For this review, take the finished solid that the model builds, in its own axes (mm). A direction names the side the tool comes from. Give positions to 0.01 mm unless a question says otherwise; leave off trailing zeros. Write each loop counter-clockwise with the first axis right and the second up, starting at its lowest first coordinate (ties: lowest second). Pieces come first, ordered by that corner, then holes. Notation, with made-up numbers: (7, 75.25) -> (27, 75.25) arc R13 cw to (27, 92.25) -> close; hole circle Ø7 at (60.25, 53). An arc over 180 degrees is marked (long way). Answer as CSV lines item,"result".
```python
from build123d import *

# Parameters (mm, degrees)
SKETCH2_R            = 215
SKETCH2_R_2          = 190
SKETCH2_R_3          = 155
BOSS_EXTRUDE1_DEPTH  = 390
SKETCH2_3_R          = 155
SKETCH2_3_R_2        = 125
BOSS_EXTRUDE2_DEPTH  = 315
SKETCH2_5_R          = 125
SKETCH2_5_R_2        = 105
SKETCH2_5_R_3        = 80
BOSS_EXTRUDE4_DEPTH  = 190
SKETCH2_6_R          = 125
SKETCH2_6_R_2        = 105
SKETCH2_6_R_3        = 80
CUT_EXTRUDE1_DEPTH   = 165
SKETCH2_7_R          = 125
SKETCH2_7_R_2        = 105
BOSS_EXTRUDE5_DEPTH  = 165
CUT_EXTRUDE2_START   = -165
SKETCH2_9_R          = 105
CUT_EXTRUDE2_DEPTH   = 165
CUT_EXTRUDE2_DRAFT   = -8.7461623
SKETCH2_10_R         = 155
SKETCH2_10_R_2       = 125
BOSS_EXTRUDE6_DEPTH  = 165
SKETCH2_12_R         = 215
SKETCH2_12_R_2       = 190
CUT_EXTRUDE3_DEPTH   = 60
SKETCH2_13_R         = 290
SKETCH2_13_R_2       = 190
SKETCH2_13_R_3       = 125
SKETCH2_13_R_4       = 80
BOSS_EXTRUDE7_DEPTH  = 35
BOSS_EXTRUDE8_START  = 100
SKETCH3_R            = 190
SKETCH3_R_2          = 175
SKETCH3_R_3          = 155
SKETCH3_R_4          = 125
BOSS_EXTRUDE8_DEPTH  = 100
BOSS_EXTRUDE10_START = 150
SKETCH3_5_R          = 175
SKETCH3_5_R_2        = 155
SKETCH3_5_R_3        = 125
BOSS_EXTRUDE10_DEPTH = 150
BOSS_EXTRUDE11_START = 250
SKETCH3_6_R          = 155
SKETCH3_6_R_2        = 125
BOSS_EXTRUDE11_DEPTH = 250
CUT_EXTRUDE5_REACH   = 567.951
SKETCH4_R            = 24
CIRPATTERN2_COUNT    = 8
SKETCH6_W            = 22
SKETCH6_H            = 75
BOSS_EXTRUDE12_DEPTH = 12.5
CIRPATTERN3_COUNT    = 8


with BuildPart() as part:
    # Sketch2 → Boss-Extrude1 (new body)
    # profile 1 of 2: a face of its own
    with BuildSketch(Plane(origin=(0, 0, 0), x_dir=(0, 1, 0), z_dir=(0, 0, 1))):
        with Locations(Location((0, 0, 0), (0, 0, 270))):
            Circle(SKETCH2_R)
        Circle(SKETCH2_R_2, mode=Mode.SUBTRACT)
    # profile 2 of 2: a face of its own
    with BuildSketch(Plane(origin=(0, 0, 0), x_dir=(0, 1, 0), z_dir=(0, 0, 1))):
        Circle(SKETCH2_R_2)
        with Locations(Location((0, 0, 0), (0, 0, 270))):
            Circle(SKETCH2_R_3, mode=Mode.SUBTRACT)
    extrude(amount=-BOSS_EXTRUDE1_DEPTH)

    # Sketch2_3 → Boss-Extrude2 (add)
    with BuildSketch(Plane(origin=(0, 0, 0), x_dir=(0, 1, 0), z_dir=(0, 0, 1))):
        with Locations(Location((0, 0, 0), (0, 0, 270))):
            Circle(SKETCH2_3_R)
        with Locations(Location((0, 0, 0), (0, 0, 270))):
            Circle(SKETCH2_3_R_2, mode=Mode.SUBTRACT)
    extrude(amount=-BOSS_EXTRUDE2_DEPTH)

    # Sketch2_5 → Boss-Extrude4 (add)
    # profile 1 of 2: a face of its own
    with BuildSketch(Plane(origin=(0, 0, 0), x_dir=(0, 1, 0), z_dir=(0, 0, 1))):
        with Locations(Location((0, 0, 0), (0, 0, 270))):
            Circle(SKETCH2_5_R)
        Circle(SKETCH2_5_R_2, mode=Mode.SUBTRACT)
    # profile 2 of 2: a face of its own
    with BuildSketch(Plane(origin=(0, 0, 0), x_dir=(0, 1, 0), z_dir=(0, 0, 1))):
        Circle(SKETCH2_5_R_2)
        with Locations(Location((0, 0, 0), (0, 0, 270))):
            Circle(SKETCH2_5_R_3, mode=Mode.SUBTRACT)
    extrude(amount=-BOSS_EXTRUDE4_DEPTH)

    # Sketch2_6 → Cut-Extrude1 (cut)
    # profile 1 of 2: a face of its own
    with BuildSketch(Plane(origin=(0, 0, 0), x_dir=(0, 1, 0), z_dir=(0, 0, 1))):
        with Locations(Location((0, 0, 0), (0, 0, 270))):
            Circle(SKETCH2_6_R)
        Circle(SKETCH2_6_R_2, mode=Mode.SUBTRACT)
    # profile 2 of 2: a face of its own
    with BuildSketch(Plane(origin=(0, 0, 0), x_dir=(0, 1, 0), z_dir=(0, 0, 1))):
        Circle(SKETCH2_6_R_2)
        with Locations(Location((0, 0, 0), (0, 0, 270))):
            Circle(SKETCH2_6_R_3, mode=Mode.SUBTRACT)
    extrude(amount=-CUT_EXTRUDE1_DEPTH, mode=Mode.SUBTRACT)

    # Sketch2_7 → Boss-Extrude5 (add)
    with BuildSketch(Plane(origin=(0, 0, 0), x_dir=(0, 1, 0), z_dir=(0, 0, 1))):
        with Locations(Location((0, 0, 0), (0, 0, 270))):
            Circle(SKETCH2_7_R)
        with Locations(Location((0, 0, 0), (0, 0, 270))):
            Circle(SKETCH2_7_R_2, mode=Mode.SUBTRACT)
    extrude(amount=-BOSS_EXTRUDE5_DEPTH)


with BuildPart() as cut_extrude2_tool:
    # Sketch2_9 → Cut-Extrude2 (with draft: the straight prism first)
    with BuildSketch(Plane(origin=(0, 0, 0), x_dir=(0, 1, 0), z_dir=(0, 0, 1)).offset(CUT_EXTRUDE2_START)):
        Circle(SKETCH2_9_R)
    extrude(amount=CUT_EXTRUDE2_DEPTH)
    # Cut-Extrude2: the draft: its side faces are tilted about the plane it starts from
    cut_extrude2_sides = [cut_extrude2_tool.faces().sort_by_distance(p)[0] for p in [
        (0, -105, -82.5),
    ]]
    draft(cut_extrude2_sides, Plane(origin=(0, 0, 0), x_dir=(0, 1, 0), z_dir=(0, 0, 1)).offset(CUT_EXTRUDE2_START), CUT_EXTRUDE2_DRAFT)


with BuildPart() as part_1:
    add(part.part)

    # Cut-Extrude2: cut by cut_extrude2_tool
    add(cut_extrude2_tool.part, mode=Mode.SUBTRACT)

    # Sketch2_10 → Boss-Extrude6 (add)
    with BuildSketch(Plane(origin=(0, 0, 0), x_dir=(0, 1, 0), z_dir=(0, 0, 1))):
        with Locations(Location((0, 0, 0), (0, 0, 270))):
            Circle(SKETCH2_10_R)
        with Locations(Location((0, 0, 0), (0, 0, 270))):
            Circle(SKETCH2_10_R_2, mode=Mode.SUBTRACT)
    extrude(amount=-BOSS_EXTRUDE6_DEPTH)

    # Sketch2_12 → Cut-Extrude3 (cut)
    with BuildSketch(Plane(origin=(0, 0, 0), x_dir=(0, 1, 0), z_dir=(0, 0, 1))):
        with Locations(Location((0, 0, 0), (0, 0, 270))):
            Circle(SKETCH2_12_R)
        with Locations(Location((0, 0, 0), (0, 0, 270))):
            Circle(SKETCH2_12_R_2, mode=Mode.SUBTRACT)
    extrude(amount=-CUT_EXTRUDE3_DEPTH, mode=Mode.SUBTRACT)

    # Sketch2_13 → Boss-Extrude7 (add)
    # profile 1 of 2: a face of its own
    with BuildSketch(Plane(origin=(0, 0, 0), x_dir=(0, 1, 0), z_dir=(0, 0, 1))):
        with Locations(Location((0, 0, 0), (0, 0, 270))):
            Circle(SKETCH2_13_R)
        with Locations(Location((0, 0, 0), (0, 0, 270))):
            Circle(SKETCH2_13_R_2, mode=Mode.SUBTRACT)
    # profile 2 of 2: a face of its own
    with BuildSketch(Plane(origin=(0, 0, 0), x_dir=(0, 1, 0), z_dir=(0, 0, 1))):
        with Locations(Location((0, 0, 0), (0, 0, 270))):
            Circle(SKETCH2_13_R_3)
        with Locations(Location((0, 0, 0), (0, 0, 270))):
            Circle(SKETCH2_13_R_4, mode=Mode.SUBTRACT)
    extrude(amount=-BOSS_EXTRUDE7_DEPTH)

    # Sketch3 → Boss-Extrude8 (add)
    # profile 1 of 3: a face of its own
    with BuildSketch(Plane.XY.offset(BOSS_EXTRUDE8_START)):
        Circle(SKETCH3_R)
        Circle(SKETCH3_R_2, mode=Mode.SUBTRACT)
    # profile 2 of 3: a face of its own
    with BuildSketch(Plane.XY.offset(BOSS_EXTRUDE8_START)):
        Circle(SKETCH3_R_2)
        Circle(SKETCH3_R_3, mode=Mode.SUBTRACT)
    # profile 3 of 3: a face of its own
    with BuildSketch(Plane.XY.offset(BOSS_EXTRUDE8_START)):
        Circle(SKETCH3_R_3)
        Circle(SKETCH3_R_4, mode=Mode.SUBTRACT)
    extrude(amount=-BOSS_EXTRUDE8_DEPTH)

    # Sketch3_5 → Boss-Extrude10 (add)
    # profile 1 of 2: a face of its own
    with BuildSketch(Plane.XY.offset(BOSS_EXTRUDE10_START)):
        Circle(SKETCH3_5_R)
        Circle(SKETCH3_5_R_2, mode=Mode.SUBTRACT)
    # profile 2 of 2: a face of its own
    with BuildSketch(Plane.XY.offset(BOSS_EXTRUDE10_START)):
        Circle(SKETCH3_5_R_2)
        Circle(SKETCH3_5_R_3, mode=Mode.SUBTRACT)
    extrude(amount=-BOSS_EXTRUDE10_DEPTH)

    # Sketch3_6 → Boss-Extrude11 (add)
    with BuildSketch(Plane.XY.offset(BOSS_EXTRUDE11_START)):
        Circle(SKETCH3_6_R)
        Circle(SKETCH3_6_R_2, mode=Mode.SUBTRACT)
    extrude(amount=-BOSS_EXTRUDE11_DEPTH)

    # Sketch4 → Cut-Extrude5 (cut, up to next)
    with BuildSketch(Plane.XY, mode=Mode.PRIVATE) as cut_extrude5_sk1:
        with Locations((221.731087803, 91.844023768)):
            Circle(SKETCH4_R)
    cut_extrude5_tool1 = extrude(cut_extrude5_sk1.sketch, amount=-CUT_EXTRUDE5_REACH, mode=Mode.PRIVATE) & part_1.part
    cut_extrude5 = cut_extrude5_tool1.solids().sort_by_distance((221.731088, 91.844024, 0))[0]
    add(cut_extrude5, mode=Mode.SUBTRACT)

    # CirPattern2: Cut-Extrude5 ×8 about axis
    cirpattern2_axis = Axis((0, 0, 0), (0, 0, 1))
    for i in range(1, CIRPATTERN2_COUNT):
        add(cut_extrude5.rotate(cirpattern2_axis, i * 360 / CIRPATTERN2_COUNT), mode=Mode.SUBTRACT)

    # Sketch6 → Boss-Extrude12 (add, symmetric)
    with BuildSketch(Plane.YZ):
        Polygon((-190, 0), (-264, 0), (-190, 75), align=None)
        with Locations((-179, 37.5)):
            Rectangle(SKETCH6_W, SKETCH6_H)
    boss_extrude12 = extrude(amount=BOSS_EXTRUDE12_DEPTH, both=True)

    # CirPattern3: Boss-Extrude12 ×8 about axis
    cirpattern3_axis = Axis((0, 0, 0), (0, 0, 1))
    for i in range(1, CIRPATTERN3_COUNT):
        add(boss_extrude12.rotate(cirpattern3_axis, i * 360 / CIRPATTERN3_COUNT))


solid = part_1.part
```
Q1. Add section B-B (y = 227). Write out the cut boundary in (x, z).
Answer block:
outline,"(-180.47, -35) -> (-115.26, -35) -> (-115.26, 0) -> (-180.47, 0) -> close; (-68.43, -35) -> (68.43, -35) -> (68.43, 0) -> (12.5, 0) -> (12.5, 37.5) -> (-12.5, 37.5) -> (-12.5, 0) -> (-68.43, 0) -> close; (115.26, -35) -> (180.47, -35) -> (180.47, 0) -> (115.26, 0) -> close"
Q2. To check wall thickness, follow probe 1 along Z at (x, y) = (-0.5, 104); probe 2 along Z at (x, y) = (-209.5, 26.5); probe 3 along X at (y, z) = (220.5, -31). State the ranges of each line that lie inside material, in increasing order. Write a range as [from, to].
Answer block:
probe 1,"z = [-190, -165], [-35, 0]"
probe 2,"z = [-390, -60], [-35, 0]"
probe 3,"x = [-188.36, -115.81], [-67.88, 67.88], [115.81, 188.36]"
Q3. Draft analysis for pull direction Z (two halves, no side actions). For faces 1 (the conical face through (-33.83, 107.44, -115.35)), 2 (the flat face through (82, -2, -190)), 3 (the flat face through (218, -12.5, 30)), 4 (the flat face through (-161.003, 160.756, 36.975)), state which applies: released by +Z, released by -Z, zero draft, split by the parting line, or undercut.
Answer block:
face 1,"undercut"
face 2,"released by -Z"
face 3,"zero draft"
face 4,"released by +Z"
Q4. Clearance check with flat-ended pins moving along their axes: pin 1 (2.5 mm diameter, centred on x = -139, y = -128, fed in from +Z); pin 2 (4 mm diameter, centred on x = 102.5, z = -125, fed in from -Y); pin 3 (2 mm diameter, centred on y = 84.5, z = 81, fed in from -X). State where each tip first meets the part, or that it passes through.
Answer block:
pin 1,"stops at z = 100"
pin 2,"stops at y = -190.07"
pin 3,"stops at x = -170.67"
Q5. Add section C-C (z = 128). Write out the cut boundary in (x, y).
Answer block:
outline,"circle Ø350 at (0, 0); hole circle Ø250 at (0, 0)"
Q6. For faces 5 (the flat face through (145.31, -162.99, 29.69)), 6 (the flat face through (-104, 70, -315)), 7 (the cylindrical face through (-33.601, -151.314, 200.7)), 8 (the flat face through (60, -189, -35)), 9 (the flat face through (162.99, -145.31, 29.69)), list the 3-axis set-ups (+Z, -Z, +X, -X, +Y, -Y) from which the entire face can be reached by the end or side of a thin tool; tool diameter is ignored.
Answer block:
face 5,"+Z, -Y"
face 6,"-Z"
face 7,"+Z"
face 8,"none"
face 9,"+Z, +X"
